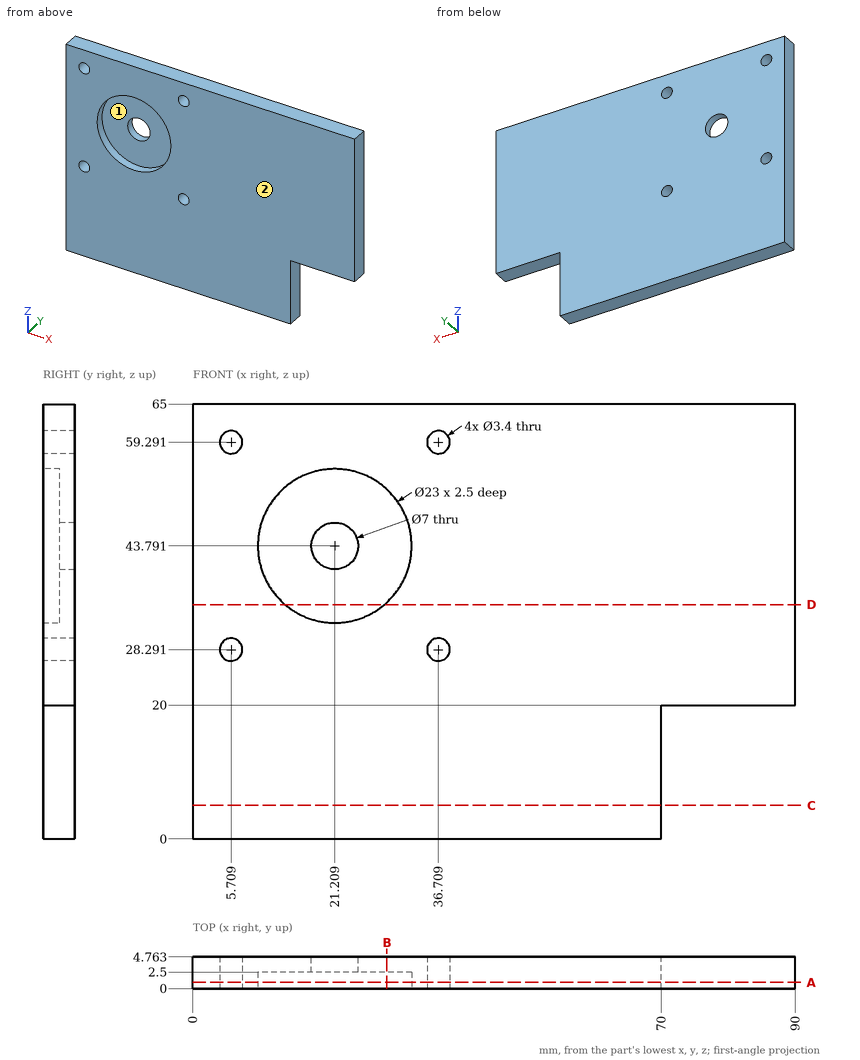
Source: three-view drawing plus pictorial views. Frame: mm from the lowest corner of the part. Coordinates: 2 decimals unless noted, no trailing zeros. Loops run counter-clockwise (first coordinate to the right, second up) from the corner with the lowest first, then second, coordinate; pieces in that order, holes last. Notation, with made-up numbers: (8, 32.5) -> (64, 32.5) arc R17 cw to (64, 50.5) -> close; hole circle Ø8 at (26.5, 33.5). An arc over 180 degrees is marked (long way). One line per item, written item: value.
(1) Cut plane C-C (z = 5). Output: boundary loops of the cut face in (x, y).
Answer below:
outline: (0, 0) -> (70, 0) -> (70, 4.76) -> (0, 4.76) -> close
(2) Draft query along X for the marked faces 1 and 2. Return one class per face: pulls with the +X half, pulls with the -X half, needs draft (parallel to the pull), parting line crosses it, or undercut.
Answer below:
face 1: undercut
face 2: needs draft
(3) Ray query, line 1 along X through (y, z) = (3.3, 59.5) (1 decimal); line 2 along Z through (x, y) = (20.5, 0.5); line 3 along Z through (x, y) = (85, 1.85). Return the intervals inside material, ascending.
Answer below:
line 1: x = 0 to 4, 7.4 to 35, 38.4 to 90
line 2: z = 0 to 32.31, 55.27 to 65
line 3: z = 20 to 65
(4) Pin query (flat end, axial travel): pin 1 Ø9 at (x, z) = (21.209, 43.791) entering from -Y; pin 2 Ø3 at (x, z) = (5.709, 28.291) entering from +Y; pin 3 Ø2.5 at (y, z) = (2.5, 14) entering from +X. Return the tip coordinate at first contact, or that it passes through.
Answer below:
pin 1: stops at y = 2.5
pin 2: passes through
pin 3: stops at x = 70
(5) Cut plane D-D (z = 35). Output: boundary loops of the cut face in (x, y) (1 decimal).
Answer below:
outline: (0, 0) -> (13.8, 0) -> (13.8, 2.5) -> (28.6, 2.5) -> (28.6, 0) -> (90, 0) -> (90, 4.8) -> (0, 4.8) -> close
(6) Cut plane A-A (y = 0.95). Output: boundary loops of the cut face in (x, z), then the cut area to 3 significant figures.
Answer below:
outline: (0, 0) -> (70, 0) -> (70, 20) -> (90, 20) -> (90, 65) -> (0, 65) -> close; hole circle Ø3.4 at (5.71, 28.29); hole circle Ø3.4 at (5.71, 59.29); hole circle Ø23 at (21.21, 43.79); hole circle Ø3.4 at (36.71, 28.29); hole circle Ø3.4 at (36.71, 59.29)
area: 5,000 mm2
(7) Cut plane B-B (x = 29). Output: boundary loops of the cut face in (y, z), then the cut area to 3 significant figures.
Answer below:
outline: (0, 0) -> (4.76, 0) -> (4.76, 65) -> (0, 65) -> (0, 52.25) -> (2.5, 52.25) -> (2.5, 35.33) -> (0, 35.33) -> close
area: 267 mm2
